For this review, use the dimensioned drawing (mm, ordinates from the lowest corner) and the shaded views. Give positions to 0.01 mm unless a question says otherwise; leave off trailing zeros. Order: outer loops, then holes, each group sorted by start corner. A loop starts at its lowest first (then second) coordinate and runs counter-clockwise, first axis right, second up. Notation, with made-up numbers: (47.25, -27) -> (106.25, -27) arc R26 ccw to (106.25, -3) -> close; hole circle Ø6 at (11.5, 43.25). An arc over 180 degrees is marked (long way). Answer as a JSON object with one key per item and string values. Group by question number.
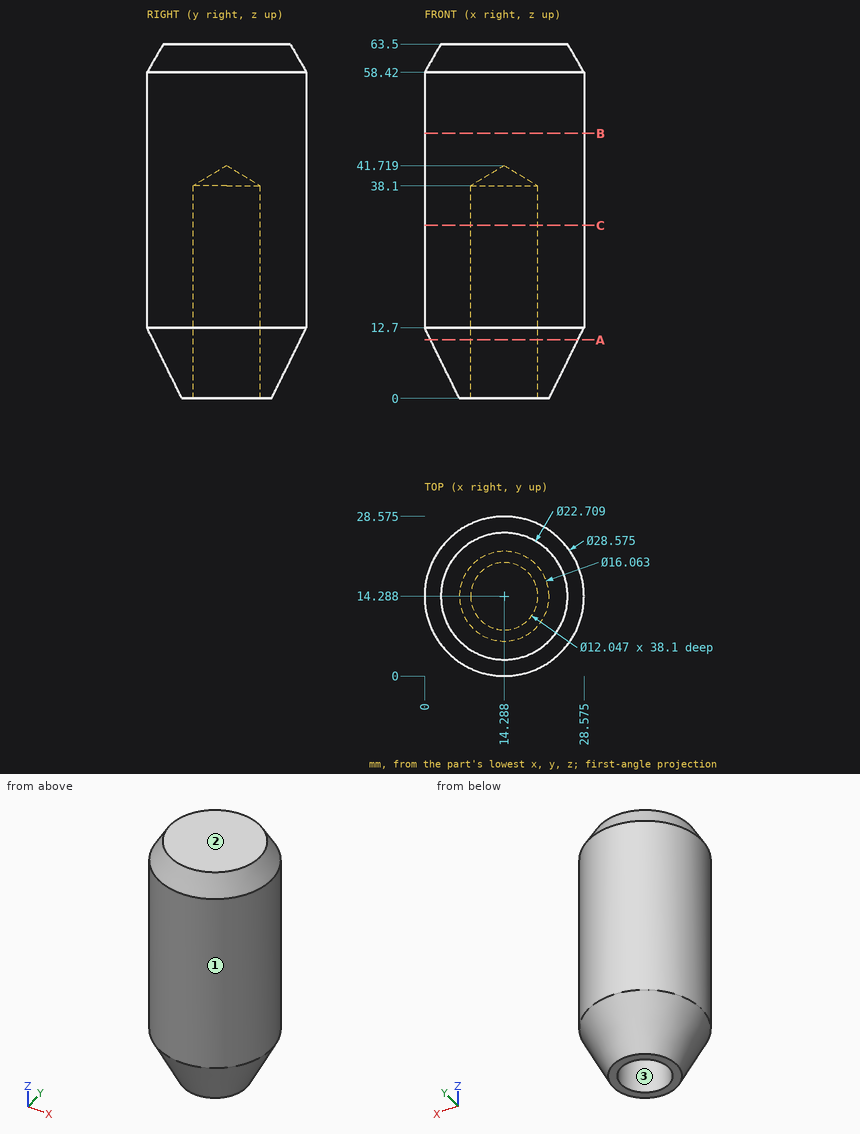
1. For pin 1 (3 mm diameter, centred on y = 22, z = 16.5, fed in from +X); pin 2 (6 mm diameter, centred on x = 14.5, y = 15, fed in from -Z); pin 3 (2 mm diameter, centred on x = 21, z = 56.5, fed in from -Y), all flat-tipped, find the tip position at first contact; note any pin that passes through.
2. Take a section at B-B on z = 47.5. Give the boundary of the cut face in (x, y) (1 decimal), plus the area to 3 significant figures.
3. For probe 1 along Y at (x, z) = (14, 31) (1 decimal); probe 2 along Z at (x, y) = (18, 23) (1 decimal); probe 3 along X at (y, z) = (12.5, 20) (1 decimal), list the stretches that pass through material, from the lowest coordinate up. Write a range as [from, to].
4. Take a section at A-A on z = 10.5. Give the boundary of the cut face in (x, y).
5. Draft analysis for pull direction X (two halves, no side actions). For the marked faces 1, 2 and 3, state which applies: pulls with the +X half, pulls with the -X half, needs draft (parallel to the pull), parting line crosses it, or undercut.
6. Take a section at C-C on z = 31. Give the boundary of the cut face in (x, y) (1 decimal), plus the area to 3 significant figures.
Checks:
{
 "1": {"pin 1": "stops at x = 27.15", "pin 2": "stops at z = 39.47", "pin 3": "stops at y = 1.19"},
 "2": {"outline": "circle Ø28.6 at (14.3, 14.3)", "area": "641 mm2"},
 "3": {"probe 1": "y = [0, 8.3], [20.3, 28.6]", "probe 2": "z = [2.9, 63.5]", "probe 3": "x = [0.1, 8.5], [20, 28.5]"},
 "4": {"outline": "circle Ø26.41 at (14.29, 14.29); hole circle Ø12.05 at (14.29, 14.29)"},
 "5": {"face 1": "parting line crosses it", "face 2": "needs draft", "face 3": "undercut"},
 "6": {"outline": "circle Ø28.6 at (14.3, 14.3); hole circle Ø12 at (14.3, 14.3)", "area": "527 mm2"}
}
